```python
from build123d import *

# Parameters (mm, degrees)
F0_R     = 50.8
F1_DEPTH = 190.5
F2_R     = 6.35
F3_DEPTH = 47.625
F4_R     = 25.4
F4_R_2   = 22.225
F5_DEPTH = 19.05
F7_DEPTH = 44.45


# Not quite as in the source:
# - a feature names something its author has since deleted; it is built from what else it names


with BuildPart() as f1:
    # F0 (on Front) → F1 (new body)
    with BuildSketch(Plane.XZ):
        Circle(F0_R)
    extrude(amount=-F1_DEPTH)

    # F2 (on face) → F3 (join)
    with BuildSketch(Plane.XZ):
        Circle(F2_R)
    extrude(amount=F3_DEPTH)

    # F4 (on face) → F5 (join)
    with BuildSketch(Plane.XZ):
        Circle(F4_R)
        Circle(F4_R_2, mode=Mode.SUBTRACT)
    extrude(amount=F5_DEPTH)

    # F6 (on face) → F7 (join)
    with BuildSketch(Plane(origin=(0, 190.5, 0), x_dir=(-1, 0, 0), z_dir=(0, 1, 0))):
        with BuildLine():
            Line((43.9940905122, 25.4), (58.1987113259, 25.4))
            ThreePointArc((58.1987113259, 25.4), (0, 63.5), (-58.1987113259, 25.4))
            Line((-58.1987113259, 25.4), (-43.9940905122, 25.4))
            ThreePointArc((-43.9940905122, 25.4), (0, 50.8), (43.9940905122, 25.4))
        make_face()
        with BuildLine():
            Line((0, 25.4), (43.9940905122, 25.4))
            ThreePointArc((43.9940905122, 25.4), (0, 50.8), (-43.9940905122, 25.4))
            Line((-43.9940905122, 25.4), (0, 25.4))
        make_face()
    extrude(amount=F7_DEPTH)


solid = f1.part
```
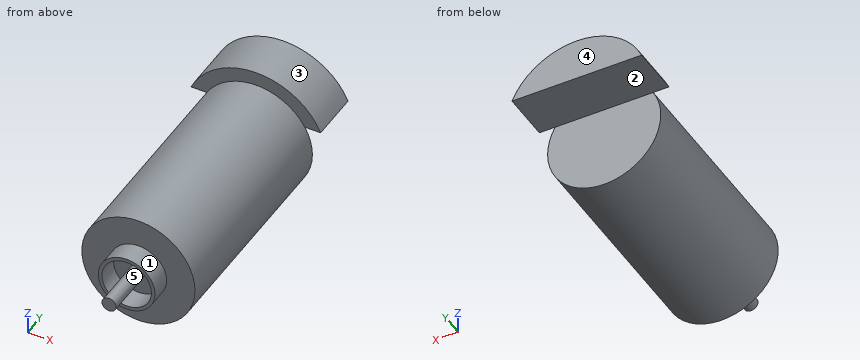
Geometry: final body of the model. Coordinates: model frame, mm. Face numbers are marked on the shaded views. A direction names the side the tool comes from. Coordinates: 2 decimals unless noted, no trailing zeros. Write each loop counter-clockwise with the first axis right and the second up, starting at its lowest first coordinate (ties: lowest second). Pieces come first, ordered by that corner, then holes. Notation, with made-up numbers: M 65,50 L 120,50 A22 ccw 120,78 Z; hole C 1.25,15 d9. An arc over 180 degrees is marked long. Answer as CSV lines item,"result". Start each with the question number.
Q1. Cut plane B-B on z = 0. Return the cut outline in (x, y) (3 decimals).
Q2. Mould query, pull axis X, two halves, no side actions, for the marked faces 3, 4 and 5. Classes: released by +X, released by -X, zero draft, split by the parting line, or undercut.
Q3. Pin query (flat end, axial travel): P1, Ø10, axis at y = 9.5, z = -1, coming from the +X side; P2, Ø4, axis at y = 87, z = -33.5, coming from the +X side; P3, Ø5, axis at x = -14.5, y = 117.5, coming from the -Z side. Return the tip coordinate at first contact, or that it passes through.
Q4. Cut plane A-A on x = 0. Return the cut outline in (y, z) (3 decimals), then the cut area to 3 significant figures.
Q5. Cut plane C-C on y = 13.5. Return the cut outline in (x, z).
Q6. Cut plane D-D on x = 32. Return the cut outline in (y, z).
Q7. Line query: line 1 (Z direction, x = 0, y = -7.25) (3 decimals); line 2 (Y direction, x = -25.5, z = -15); line 3 (Y direction, x = 1, z = 51). Output: solid intervals per line, ascending. Write a range as from..to.
Q8. Reachability of the marked faces 1 and 2 from +Z, -Z, +X, -X, +Y, -Y: full face, straight path, thin tool, end or side. Return the list, or none.
Findings below:
1,outline,"M -50.8,0 L -25.4,0 L -25.4,-19.05 L -22.225,-19.05 L -22.225,0 L -6.35,0 L -6.35,-47.625 L 6.35,-47.625 L 6.35,0 L 22.225,0 L 22.225,-19.05 L 25.4,-19.05 L 25.4,0 L 50.8,0 L 50.8,190.5 L -50.8,190.5 Z"
2,face 3,"split by the parting line"
2,face 4,"zero draft"
2,face 5,"undercut"
3,P1,"stops at x = 50.8"
3,P2,"stops at x = 39.85"
3,P3,"stops at z = -49.36"
4,outline,"M -47.625,-6.35 L 0,-6.35 L 0,-22.225 L -19.05,-22.225 L -19.05,-25.4 L 0,-25.4 L 0,-50.8 L 190.5,-50.8 L 190.5,25.4 L 234.95,25.4 L 234.95,63.5 L 190.5,63.5 L 190.5,50.8 L 0,50.8 L 0,25.4 L -19.05,25.4 L -19.05,22.225 L 0,22.225 L 0,6.35 L -47.625,6.35 Z"
4,area,"21,800 mm2"
5,outline,"C 0,0 d101.6"
6,outline,"M 0,-39.45 L 190.5,-39.45 L 190.5,25.4 L 234.95,25.4 L 234.95,54.85 L 190.5,54.85 L 190.5,39.45 L 0,39.45 Z"
7,line 1,"z = -25.4..-22.225, -6.35..6.35, 22.225..25.4"
7,line 2,"y = 0..190.5"
7,line 3,"y = 190.5..234.95"
8,face 1,"-Y"
8,face 2,"-Z, +X, -X, +Y"
